```python
from build123d import *

# Parameters (mm, degrees)
SKETCH1_R           = 3
BOSS_EXTRUDE1_DEPTH = 62
BOSS_EXTRUDE2_DEPTH = 3


with BuildPart() as part:
    # Sketch1 → Boss-Extrude1 (new body)
    with BuildSketch(Plane.XY):
        with Locations((-43.2, 0)):
            Circle(SKETCH1_R)
    extrude(amount=-BOSS_EXTRUDE1_DEPTH)

    # Sketch2 → Boss-Extrude2 (add)
    with BuildSketch(Plane.XY):
        with BuildLine():
            Line((-47.054399712, -2.442285905), (-43.212081089, -4.563004671))
            ThreePointArc((-43.212081089, -4.563004671), (-43.111583363, -4.58786779), (-43.012118219, -4.559151019))
            Line((-43.012118219, -4.559151019), (-39.254362582, -2.291964865))
            ThreePointArc((-39.254362582, -2.291964865), (-39.182581626, -2.217362841), (-39.157718507, -2.116865114))
            Line((-39.157718507, -2.116865114), (-39.242281493, 2.271039806))
            ThreePointArc((-39.242281493, 2.271039806), (-39.270998264, 2.370504949), (-39.345600288, 2.442285905))
            Line((-39.345600288, 2.442285905), (-43.187918911, 4.563004671))
            ThreePointArc((-43.187918911, 4.563004671), (-43.288416637, 4.58786779), (-43.387881781, 4.559151019))
            Line((-43.387881781, 4.559151019), (-47.145637418, 2.291964865))
            ThreePointArc((-47.145637418, 2.291964865), (-47.217418374, 2.217362841), (-47.242281493, 2.116865114))
            Line((-47.242281493, 2.116865114), (-47.157718507, -2.271039806))
            ThreePointArc((-47.157718507, -2.271039806), (-47.129001736, -2.370504949), (-47.054399712, -2.442285905))
        make_face()
    extrude(amount=BOSS_EXTRUDE2_DEPTH)


solid = part.part
```
Input: part model. Units: mm. Frame: model coordinates. A direction names the side the tool comes from. Give positions to 0.01 mm unless a question says otherwise; leave off trailing zeros. Order: outer loops, then holes, each group sorted by start corner. A loop starts at its lowest first (then second) coordinate and runs counter-clockwise, first axis right, second up.
1. Cut plane D-D (y = -4). Return loops of the section in (x, z), and give its area (3 significant figures).
Computed:
outline: (-44.23, 0) - (-42.09, 0) - (-42.09, 3) - (-44.23, 3) - close
area: 6.44 mm2
2. Cut plane A-A (x = -41.75). Return loops of the section in (y, z), and give its area (3 significant figures).
Computed:
outline: (-3.8, 0) - (-2.63, 0) - (-2.63, -62) - (2.63, -62) - (2.63, 0) - (3.77, 0) - (3.77, 3) - (-3.8, 3) - close
area: 348 mm2
3. Set-up query: faces 1 (the face through (-42, -3, 0)), 2 (the face through (-45.16, -3.49, 1.48)). Return all of +Z, -Z, +X, -X, +Y, -Y with unobstructed straight access to the full face (end or side cutting, diameter ignored); none if empty.
Computed:
face 1: -Z
face 2: +Z, -Z, -X, -Y
4. Line query: probe 1 along Z at (x, y) = (-40.5, 2.5); probe 2 along Y at (x, z) = (-40.75, -23); probe 3 along Y at (x, z) = (-43.75, -11). Output: solid intervals per line, ascending.
Computed:
probe 1: z = 0 to 3
probe 2: y = -1.73 to 1.73
probe 3: y = -2.95 to 2.95
5. Cut plane B-B (z = -29.5). Return loops of the section in (x, y), and give its area (3 significant figures).
Computed:
outline: circle Ø6 at (-43.2, 0)
area: 28.3 mm2
6. Cut plane C-C (y = 0). Return loops of the section in (x, z).
Computed:
outline: (-47.2, 0) - (-46.2, 0) - (-46.2, -62) - (-40.2, -62) - (-40.2, 0) - (-39.2, 0) - (-39.2, 3) - (-47.2, 3) - close
7. Pin query (flat end, axial travel): pin 1 Ø4 at (y, z) = (0, -3.5) entering from -X; pin 2 Ø2 at (x, y) = (-46.5, -3) entering from -Z; pin 3 Ø4 at (y, z) = (3.5, -8.5) entering from +X; pin 4 Ø4 at (x, y) = (-44.5, 3) entering from -Z. Return the tip coordinate at first contact, or that it passes through.
Computed:
pin 1: stops at x = -46.2
pin 2: stops at z = 0
pin 3: stops at x = -40.6
pin 4: stops at z = -62
